Geometry: final body of the model. Coordinates: model frame, mm. Round coordinates to 2 decimals unless told otherwise and drop trailing zeros. Answer as a JSON object with one key per item and string values.
Autodesk Inventor part; units mm, degrees
ref_plane "作業平面1" through (-9.5, -10, 1000) normal (0, 0, 1) x (1, 0, 0)
ref_plane "YZ Plane" through (0, 0, 0) normal (1, 0, 0) x (0, 1, 0)
ref_plane "XZ Plane" through (0, 0, 0) normal (0, 1, 0) x (-1, 0, 0)
ref_plane "作業平面1" through (-9.5, -10, 1000) normal (0, 0, 1) x (1, 0, 0)
sketch "スケッチ1" plane through (-9.5, -10, 1000) normal (0, 0, 1) x (1, 0, 0)
  line L0 (7.35, 18.5) -> (7.35, 20)
  line L1 (7.35, 20) -> (0, 20)
  arc A0 (0, 20) -> (-0.5, 19.5) centre (0, 19.5) ccw
  line L2 (-0.5, 19.5) -> (-0.5, 12.15)
  line L3 (-0.5, 12.15) -> (1, 12.15)
  line L4 (1, 12.15) -> (1, 14.15)
  line L5 (1, 14.15) -> (4.7, 14.15)
  line L6 (4.7, 14.15) -> (4.7, 12.15)
  line L7 (4.7, 12.15) -> (6.5, 12.15)
  line L8 (6.5, 12.15) -> (6.5, 7.85)
  line L9 (6.5, 7.85) -> (4.7, 7.85)
  line L10 (4.7, 7.85) -> (4.7, 5.85)
  line L11 (4.7, 5.85) -> (1, 5.85)
  line L12 (1, 5.85) -> (1, 7.85)
  line L13 (1, 7.85) -> (-0.5, 7.85)
  line L14 (-0.5, 7.85) -> (-0.5, 0.5)
  arc A1 (-0.5, 0.5) -> (0, 0) centre (0, 0.5) ccw
  line L15 (0, 0) -> (19, 0)
  arc A2 (19, 0) -> (19.5, 0.5) centre (19, 0.5) ccw
  line L16 (19.5, 0.5) -> (19.5, 19.5)
  arc A3 (19.5, 19.5) -> (19, 20) centre (19, 19.5) ccw
  line L17 (19, 20) -> (11.65, 20)
  line L18 (11.65, 20) -> (11.65, 18.5)
  line L19 (11.65, 18.5) -> (13.65, 18.5)
  line L20 (13.65, 18.5) -> (13.65, 14.8)
  line L21 (13.65, 14.8) -> (11.65, 14.8)
  line L22 (11.65, 14.8) -> (11.65, 13)
  line L23 (11.65, 13) -> (7.35, 13)
  line L24 (7.35, 13) -> (7.35, 14.8)
  line L25 (7.35, 14.8) -> (5.35, 14.8)
  line L26 (5.35, 14.8) -> (5.35, 18.5)
  line L27 (5.35, 18.5) -> (7.35, 18.5)
  arc A4 (17.7174, 15.4132) -> (17.6402, 15.0252) centre (17.9, 15.1752) ccw
  line L28 (17.6402, 15.0252) -> (17.9598, 14.4715)
  arc A5 (18, 14.3215) -> (17.9598, 14.4715) centre (17.7, 14.3215) ccw
  line L29 (18, 14.3215) -> (18, 6.7162)
  arc A6 (17.7225, 6.4162) -> (18, 6.7162) centre (17.7, 6.7153) ccw
  line L30 (17.7225, 6.4162) -> (17.0355, 6.4162)
  arc A7 (17.0355, 6.4162) -> (16.8233, 6.3283) centre (17.0355, 6.1162) ccw
  line L31 (16.8233, 6.3283) -> (15.9875, 5.4924)
  arc A8 (15.9875, 5.4924) -> (16.2388, 4.9829) centre (16.1996, 5.2803) ccw
  arc A9 (14.5171, 3.2612) -> (16.2388, 4.9829) centre (16.5, 3) ccw
  arc A10 (14.5171, 3.2612) -> (14.2973, 3.5902) centre (14.2197, 3.3004) ccw
  line L32 (14.2973, 3.5902) -> (14.2135, 3.6127)
  arc A11 (14.2135, 3.6127) -> (13.9237, 3.535) centre (14.1359, 3.3229) ccw
  line L33 (13.9237, 3.535) -> (13.0879, 2.6991)
  arc A12 (13.0879, 2.6991) -> (13, 2.487) centre (13.3, 2.487) ccw
  line L34 (13, 2.487) -> (13, 1.8)
  arc A13 (12.7, 1.5) -> (13, 1.8) centre (12.7, 1.8) ccw
  line L35 (12.7, 1.5) -> (5.1785, 1.5)
  arc A14 (5.0285, 1.5402) -> (5.1785, 1.5) centre (5.1785, 1.8) ccw
  line L36 (5.0285, 1.5402) -> (4.4748, 1.8598)
  arc A15 (4.4748, 1.8598) -> (4.0868, 1.7826) centre (4.3248, 1.6) ccw
  arc A16 (4.0868, 4.2174) -> (4.0868, 1.7826) centre (2.5, 3) ccw
  arc A17 (4.0868, 4.2174) -> (4.4748, 4.1402) centre (4.3248, 4.4) ccw
  line L37 (4.4748, 4.1402) -> (6.2409, 5.1598)
  arc A18 (6.3909, 5.2) -> (6.2409, 5.1598) centre (6.3909, 4.9) ccw
  line L38 (6.3909, 5.2) -> (7.05, 5.2)
  arc A19 (7.05, 5.2) -> (7.35, 5.5) centre (7.05, 5.5) ccw
  line L39 (7.35, 5.5) -> (7.35, 6.4)
  arc A20 (7.95, 7) -> (7.35, 6.4) centre (7.95, 6.4) ccw
  line L40 (7.95, 7) -> (9.2042, 7)
  arc A21 (9.2042, 7) -> (9.4163, 7.0879) centre (9.2042, 7.3) ccw
  line L41 (9.4163, 7.0879) -> (9.9752, 7.6468)
  arc A22 (9.9752, 7.6468) -> (10.0529, 7.9366) centre (9.7631, 7.8589) ccw
  line L42 (10.0529, 7.9366) -> (9.9987, 8.1389)
  arc A23 (9.9987, 8.1389) -> (9.6768, 8.3595) centre (9.7089, 8.0612) ccw
  arc A24 (11.1405, 9.8232) -> (9.6768, 8.3595) centre (9.5, 10) ccw
  arc A25 (11.1405, 9.8232) -> (11.3611, 9.5013) centre (11.4388, 9.7911) ccw
  line L43 (11.3611, 9.5013) -> (11.5634, 9.4471)
  arc A26 (11.5634, 9.4471) -> (11.8532, 9.5248) centre (11.6411, 9.7369) ccw
  line L44 (11.8532, 9.5248) -> (12.4121, 10.0837)
  arc A27 (12.4121, 10.0837) -> (12.5, 10.2958) centre (12.2, 10.2958) ccw
  line L45 (12.5, 10.2958) -> (12.5, 11.55)
  arc A28 (13.1, 12.15) -> (12.5, 11.55) centre (13.1, 11.55) ccw
  line L46 (13.1, 12.15) -> (14, 12.15)
  arc A29 (14, 12.15) -> (14.2652, 12.4701) centre (13.966, 12.4481) ccw
  line L47 (14.2652, 12.4701) -> (14.2652, 13.0488)
  arc A30 (14.3054, 13.1988) -> (14.2652, 13.0488) centre (14.5652, 13.0488) ccw
  line L48 (14.3054, 13.1988) -> (15.3598, 15.0252)
  arc A31 (15.3598, 15.0252) -> (15.2826, 15.4132) centre (15.1, 15.1752) ccw
  arc A32 (17.7174, 15.4132) -> (15.2826, 15.4132) centre (16.5, 17) ccw
  circle A33 centre (2.5, 17) radius 2
  point P0 (9.5, 10)
extrude "押し出し1" add sketch "スケッチ1" along normal blind 620
properties part number "AFST-2020-4-1000"
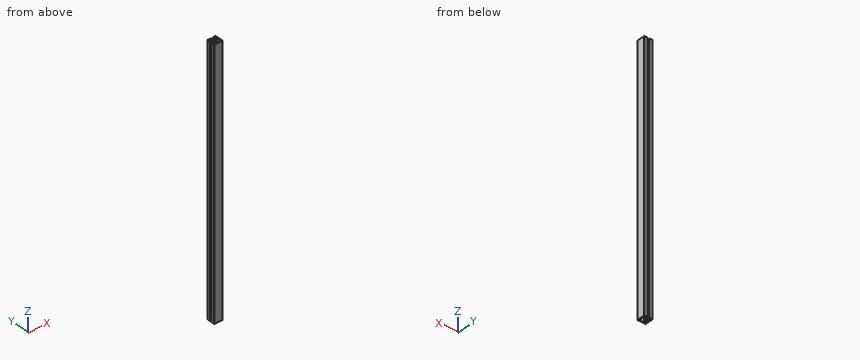
1) Ray query, line 1 (Y direction, x = 0, z = 1138.5); line 2 (Y direction, x = -7, z = 1231.5); line 3 (Y direction, x = 8.25, z = 1452). Return the intervals inside material, ascending.
Results:
{"line 1": "-10 to -8.5, -2.83 to -1.65, 1.65 to 3", "line 2": "-10 to -9, -5 to -4.15, 4.15 to 5, 9 to 10", "line 3": "-10 to -8.56, -5.44 to -3.58, 4.83 to 5.44, 8.56 to 10"}
2) Section query A-A (z = 1161.5). Count the separate pieces of the cut face and the enclosed holes in it, and give its area (3 significant figures).
Results:
{"separate pieces": "1", "enclosed holes": "2", "area": "155 mm2"}
3) Pin query (flat end, axial travel): P1, Ø3, axis at x = -7, y = 7, coming from the -Z side. Return the tip coordinate at first contact, or that it passes through.
Results:
{"P1": "through"}
